from build123d import *

# Parameters (mm, degrees)
F0_W     = 5
F0_H     = 8.571429
F1_DEPTH = 7.75
F3_DEPTH = 3.95
F5_DEPTH = 25
F6_W     = 1.201827
F6_H     = 7.746514
F7_DEPTH = 6
F8_DEPTH = 6


with BuildPart() as f1:
    # F0 (on Front) → F1 (new body)
    with BuildSketch(Plane.XZ):
        with Locations((1.341188, -1.791949)):
            Rectangle(F0_W, F0_H)
        Polygon((18.641188, -3.961869), (3.841188, 2.493765), (3.841188, -6.077664), (3.841188, -6.111869), (18.641188, -6.111869), align=None)
    extrude(amount=F1_DEPTH)

    # F2 (on Top) → F3 (join)
    with BuildSketch(Plane.XY):
        with BuildLine():
            ThreePointArc((-0.070193, -4.217616), (1.020355, -5.308165), (2.110904, -4.217616))
            ThreePointArc((2.110904, -4.217616), (1.020355, -3.127068), (-0.070193, -4.217616))
        make_face()
    extrude(amount=F3_DEPTH)

    # F4 (on Top) → F5 (cut)
    with BuildSketch(Plane.XY):
        Polygon((0, -1.442116), (0, -6.315767), (2.538758, -6.315767), (2.538758, -1.442116), (1.405665, -1.442116), align=None)
    extrude(amount=-F5_DEPTH, mode=Mode.SUBTRACT)

    # F6 (on Top) → F7 (join)
    with BuildSketch(Plane.XY):
        with Locations((3.216505, -3.873257)):
            Rectangle(F6_W, F6_H)
    extrude(amount=-F7_DEPTH)

    # F6 (on Top) → F8 (join)
    with BuildSketch(Plane.XY):
        with Locations((3.216505, -3.873257)):
            Rectangle(F6_W, F6_H)
    extrude(amount=-F8_DEPTH)


solid = f1.part
Could you check a few things on this model? Use its own coordinates, in mm. A direction names the side the tool comes from. Coordinates: 2 decimals unless noted, no trailing zeros. Loops run counter-clockwise (first coordinate to the right, second up) from the corner with the lowest first, then second, coordinate; pieces in that order, holes last.
1. Imagine slicing it at D-D (z = 1). Please give me the cut outline in (x, y), and give its area (3 significant figures).
2. Imagine slicing it at C-C (x = 3.5). Please give me the cut outline in (y, z).
3. Imagine slicing it at A-A (z = -2.5). Please give me the cut outline in (x, y), and give its area (3 significant figures).
4. For P1, Ø2.5, axis at y = -4.5, z = -2, coming from the +X side; P2, Ø4, axis at x = 1.5, y = -5, coming from the -Z side; P3, Ø1, axis at y = -7, z = -3, coming from the +X side, each with a flat end and sliding along its axis, tell me the tip position at first contact or that it passes through.
5. For faces 1 (the face through (-0.4, -3.8, -6.078)), 2 (the face through (2.539, -4, -3)), 3 (the face through (0.2, -3.5, 3.2)), 4 (the face through (1, -4, 3.95)), which set-ups out of +Z, -Z, +X, -X, +Y, -Y let a thin tool reach every point of the face, with its end or its side?
6. I need wall thicknesses on L1, parallel to X at y = -4, z = -5.5; L2, parallel to Z at x = 3, y = -6.5; L3, parallel to X at y = -2.25, z = -0.25. Which ranges of each line are inside material? Lowest first, please.
7. We'd pull the mould along X, two halves only. Please class faces 5 (the face through (1, -4, 0)), 6 (the face through (-1.159, -4, -2)), 7 (the face through (6, -7.75, -3)): released by +X, released by -X, zero draft, split by the parting line, or undercut.
Computed values:
1. outline: (-1.16, -7.75) - (7.27, -7.75) - (7.27, 0) - (-1.16, 0) - close
1. area: 65.3 mm2
2. outline: (-7.75, -6.08) - (0, -6.08) - (0, 2.49) - (-7.75, 2.49) - close
3. outline: (-1.16, -7.75) - (15.29, -7.75) - (15.29, 0) - (-1.16, 0) - close; hole (0, -6.32) - (2.54, -6.32) - (2.54, -1.44) - (0, -1.44) - close
3. area: 115 mm2
4. P1: stops at x = 17.01
4. P2: stops at z = -6.08
4. P3: stops at x = 17.58
5. face 1: -Z, -X, +Y, -Y
5. face 2: -Z
5. face 3: +Z
5. face 4: +Z, +X, -X, +Y, -Y
6. L1: x = -1.16 to 0, 2.54 to 18.64
6. L2: z = -6.08 to 2.49
6. L3: x = -1.16 to 0, 2.54 to 10.13
7. face 5: undercut
7. face 6: released by -X
7. face 7: zero draft
